Can you work these out from the model? Positions are in its coordinate system, mm. Round coordinates to 2 decimals unless told otherwise and drop trailing zeros. Answer as a JSON object with one key per item and string values.
```python
from build123d import *

# Parameters (mm, degrees)
MODEL_R                 = 1.5
SALIENTE_EXTRUIR1_DEPTH = 3


with BuildPart() as part:
    # Model → Saliente-Extruir1 (new body)
    with BuildSketch(Plane.XY):
        with BuildLine():
            Line((213.25077615, 71.428489513), (213.25077615, 188.428489513))
            ThreePointArc((213.25077615, 188.428489513), (208.75077615, 192.928489513), (204.25077615, 188.428489513))
            Line((204.25077615, 188.428489513), (204.25077615, 71.428489513))
            ThreePointArc((204.25077615, 71.428489513), (208.75077615, 66.928489513), (213.25077615, 71.428489513))
        make_face()
        with Locations((208.75077615, 179.428489513)):
            Circle(MODEL_R, mode=Mode.SUBTRACT)
        with Locations((208.75077615, 188.428489513)):
            Circle(MODEL_R, mode=Mode.SUBTRACT)
        with Locations((208.75077615, 152.428489513)):
            Circle(MODEL_R, mode=Mode.SUBTRACT)
        with Locations((208.75077615, 161.428489513)):
            Circle(MODEL_R, mode=Mode.SUBTRACT)
        with Locations((208.75077615, 170.428489513)):
            Circle(MODEL_R, mode=Mode.SUBTRACT)
        with Locations((208.75077615, 143.428489513)):
            Circle(MODEL_R, mode=Mode.SUBTRACT)
        with Locations((208.75077615, 116.428489513)):
            Circle(MODEL_R, mode=Mode.SUBTRACT)
        with Locations((208.75077615, 125.428489513)):
            Circle(MODEL_R, mode=Mode.SUBTRACT)
        with Locations((208.75077615, 134.428489513)):
            Circle(MODEL_R, mode=Mode.SUBTRACT)
        with Locations((208.75077615, 71.428489513)):
            Circle(MODEL_R, mode=Mode.SUBTRACT)
        with Locations((208.75077615, 80.428489513)):
            Circle(MODEL_R, mode=Mode.SUBTRACT)
        with Locations((208.75077615, 89.428489513)):
            Circle(MODEL_R, mode=Mode.SUBTRACT)
        with Locations((208.75077615, 98.428489513)):
            Circle(MODEL_R, mode=Mode.SUBTRACT)
        with Locations((208.75077615, 107.428489513)):
            Circle(MODEL_R, mode=Mode.SUBTRACT)
    extrude(amount=SALIENTE_EXTRUIR1_DEPTH)


solid = part.part
```
Q1. We'd pull the mould along X, two halves only. Please class faces 1 (the flat face through (209, 131, 0)), 2 (the cylindrical face through (207.645, 162.442, 1.479)), 3 (the flat face through (213.251, 129, 1)): pulls with the +X half, pulls with the -X half, needs draft (parallel to the pull), parting line crosses it, or undercut.
Determined:
{"face 1": "needs draft", "face 2": "undercut", "face 3": "pulls with the +X half"}
Q2. I want a section at A-A, the plane z = 2.5. Give the number of separate pieces and of enclosed holes in the cut face, then the cut area to 3 significant figures.
Determined:
{"separate pieces": "1", "enclosed holes": "14", "area": "1,020 mm²"}
Q3. If I drill on L1, parallel to X at y = 144.5, z = 0.3; L2, parallel to Y at x = 205.5, z = 2.5; L3, parallel to Y at x = 210.75, z = 2.85, over which ranges is the centre line in solid material (lowest first)? Write a range as [from, to].
Determined:
{"L1": "[204.25, 207.7], [209.8, 213.25]", "L2": "[68.32, 191.54]", "L3": "[67.4, 192.46]"}
